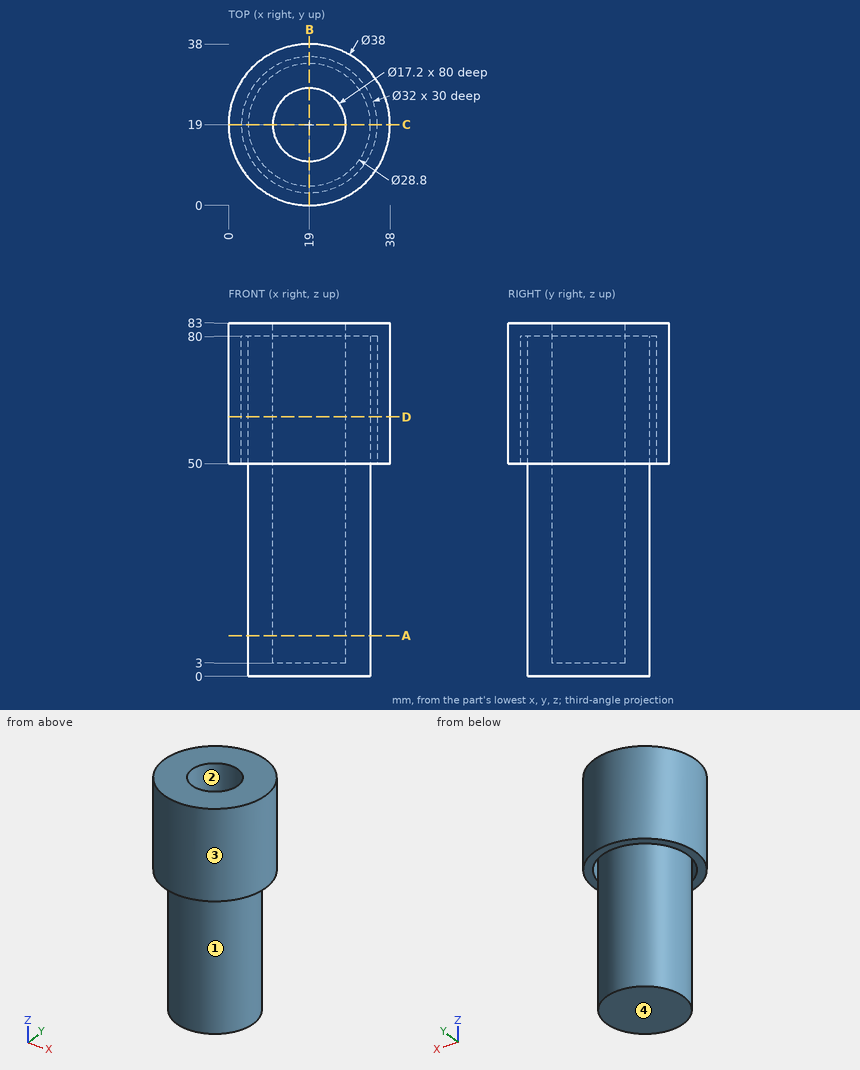
Geometry: see drawing. Coordinates: mm, zero at the bounding-box minimum. Give positions to 0.01 mm unless a question says otherwise; leave off trailing zeros. Write each loop counter-clockwise with the first axis right and the second up, starting at its lowest first coordinate (ties: lowest second). Pieces come first, ordered by that corner, then holes. Notation, with made-up numbers: M -9.75,48.5 L 1.25,48.5 A13 ccw 1.25,55.5 Z; hole C 75,1 d3. An arc over 180 degrees is marked long. Answer in a Markdown table with one row per item. Add a question column.
(1) Section D-D on z = 61. Return loops of the section in (x, y).
(2) Ray query, line 1 (Y direction, x = 19, z = 61); line 2 (Y direction, x = 19, z = 45); line 3 (Z direction, x = 22, y = 3). Return the intervals inside material, ascending.
(3) Mould query, pull axis Y, two halves, no side actions, for the marked faces 1, 2, 3 and 4. Classes: +Y half, -Y half, draft (parallel to the pull), parting line (faces both ways), or undercut.
(4) First-contact query: pin 1 (10 mm diameter, centred on x = 32, z = 59.5, fed in from +Y); pin 2 (8 mm diameter, centred on y = 7.5, z = 62.5, fed in from +X); pin 3 (1.5 mm diameter, centred on y = 20.5, z = 42.5, fed in from +X). Flat tips, straight axial feed; report the tip coordinate or a pass-through.
(5) Section B-B on x = 19. Return loops of the section in (y, z).
(6) Section A-A on z = 9.5. Return loops of the section in (x, y), and give its area (3 significant figures).
Result set:
| question | item | result |
|---|---|---|
| 1 | outline | C 19,19 d38; C 19,19 d28.8; hole C 19,19 d32; hole C 19,19 d17.2 |
| 2 | line 1 | y = 0 to 3, 4.6 to 10.4, 27.6 to 33.4, 35 to 38 |
| 2 | line 2 | y = 4.6 to 10.4, 27.6 to 33.4 |
| 2 | line 3 | z = 50 to 83 |
| 3 | face 1 | undercut |
| 3 | face 2 | undercut |
| 3 | face 3 | parting line |
| 3 | face 4 | draft |
| 4 | pin 1 | stops at y = 36.23 |
| 4 | pin 2 | stops at x = 36.46 |
| 4 | pin 3 | stops at x = 33.38 |
| 5 | outline | M 0,50 L 3,50 L 3,80 L 4.6,80 L 4.6,0 L 33.4,0 L 33.4,80 L 35,80 L 35,50 L 38,50 L 38,83 L 27.6,83 L 27.6,3 L 10.4,3 L 10.4,83 L 0,83 Z |
| 6 | outline | C 19,19 d28.8; hole C 19,19 d17.2 |
| 6 | area | 419 mm^2 |
